```python
from build123d import *

# Parameters (mm, degrees)
SKETCH_1_W          = 28
SKETCH_1_H          = 10
SKETCH_1_R          = 1.65
SKETCH_1_R_2        = 1.6
EXTRUDE_1_DEPTH     = 10
SKETCH_2_R          = 1.65
CUT_EXTRUDE_1_DEPTH = 28
SKETCH_3_W          = 10
SKETCH_3_H          = 10
SKETCH_3_R          = 1.6
CUT_EXTRUDE_2_DEPTH = 7
FILLET_1_R          = 1


with BuildPart() as part:
    # ｽｹｯﾁ1 → ﾎﾞｽ - 押し出し1 (new body)
    with BuildSketch(Plane.XY):
        with Locations((-9, 0)):
            Rectangle(SKETCH_1_W, SKETCH_1_H)
        Circle(SKETCH_1_R, mode=Mode.SUBTRACT)
        with Locations((-18, 0)):
            Circle(SKETCH_1_R_2, mode=Mode.SUBTRACT)
    extrude(amount=EXTRUDE_1_DEPTH)

    # ｽｹｯﾁ2 → ｶｯﾄ - 押し出し1 (cut, through all)
    with BuildSketch(Plane(origin=(0, 5, 0), x_dir=(1, 0, 0), z_dir=(0, 1, 0))):
        with Locations(Location((-7.5, -5, 0), (0, 0, 270))):
            Circle(SKETCH_2_R)
    extrude(amount=-CUT_EXTRUDE_1_DEPTH, mode=Mode.SUBTRACT)

    # ｽｹｯﾁ3 → ｶｯﾄ - 押し出し2 (cut)
    with BuildSketch(Plane(origin=(0, 0, 0), x_dir=(-1, 0, 0), z_dir=(0, 0, -1))):
        with Locations((18, 0)):
            Rectangle(SKETCH_3_W, SKETCH_3_H)
        with Locations((18, 0)):
            Circle(SKETCH_3_R, mode=Mode.SUBTRACT)
    extrude(amount=-CUT_EXTRUDE_2_DEPTH, mode=Mode.SUBTRACT)

    # ﾌｨﾚｯﾄ1
    fillet_1_edges = [part.edges().sort_by_distance(p)[0] for p in [
        (-13, -5, 3.5),
        (-13, 5, 3.5),
        (5, -5, 5),
        (-23, -5, 8.5),
        (-23, 5, 8.5),
        (5, 5, 5),
    ]]
    fillet(fillet_1_edges, radius=FILLET_1_R)


solid = part.part
```
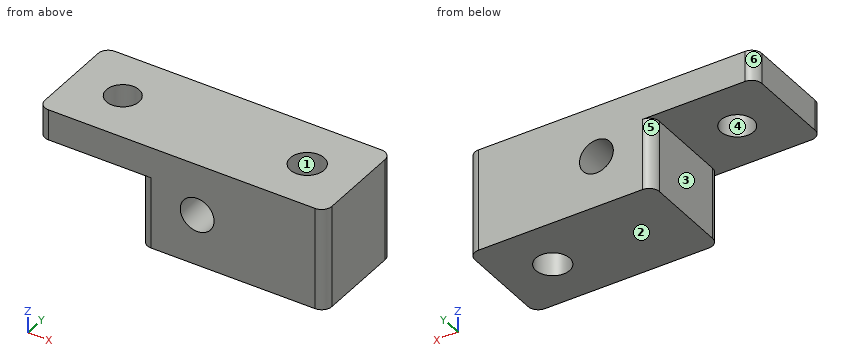
Check sheet for the modelled part. Datum: model origin and axes. Units: mm. Face numbers are marked on the shaded views. A direction names the side the tool comes from. Round coordinates to 2 decimals unless told otherwise and drop trailing zeros. Order: outer loops, then holes, each group sorted by start corner. A loop starts at its lowest first (then second) coordinate and runs counter-clockwise, first axis right, second up. Notation, with made-up numbers: (15, 59) - (51, 59) arc R18 ccw to (51, 90) - close; hole circle Ø6 at (55.25, -32). An arc over 180 degrees is marked (long way). Write item = value, one per line.
Q1. Section check D-D (z = 7.5). Record the boundary of the cut face in (x, y), and give its area (3 significant figures).
Computed:
outline = (-23, -4) arc R1 ccw to (-22, -5) - (4, -5) arc R1 ccw to (5, -4) - (5, 4) arc R1 ccw to (4, 5) - (-22, 5) arc R1 ccw to (-23, 4) - close; hole circle Ø3.2 at (-18, 0); hole circle Ø3.3 at (0, 0)
area = 263 mm^2
Q2. Go/stop test with a flat-tipped pin: pin 1 (3 mm diameter, centred on y = 0, z = 4, fed in from -X). Record where the tip stops, or that it passes through.
Computed:
pin_1 = -13
Q3. Section check A-A (z = 5). Record the boundary of the cut face in (x, y), and give its area (3 significant figures).
Computed:
outline = (-13, -4) arc R1 ccw to (-12, -5) - (-9.15, -5) - (-9.15, 5) - (-12, 5) arc R1 ccw to (-13, 4) - close; (-5.85, -5) - (4, -5) arc R1 ccw to (5, -4) - (5, 4) arc R1 ccw to (4, 5) - (-5.85, 5) - close; hole circle Ø3.3 at (0, 0)
area = 138 mm^2
Q4. Thickness scan on line 1 along X through (y, z) = (-2, 5); line 2 along X through (y, z) = (-1.25, 5); line 3 along Z through (x, y) = (-16.25, -2.5). Record the ranges inside material, lowest first.
Computed:
line_1 = -13 to -9.15, -5.85 to 5
line_2 = -13 to -9.15, -5.85 to -1.08, 1.08 to 5
line_3 = 7 to 10
Q5. Draft check along X on the marked faces 1, 2, 3 and 4. Enter one of: pulls with the +X half, pulls with the -X half, needs draft (parallel to the pull), parting line crosses it, or undercut.
Computed:
face_1 = undercut
face_2 = needs draft
face_3 = pulls with the -X half
face_4 = undercut
Q6. Section check B-B (x = 0). Record the boundary of the cut face in (y, z), and give its area (3 significant figures).
Computed:
outline = (-5, 0) - (-1.65, 0) - (-1.65, 10) - (-5, 10) - close; (1.65, 0) - (5, 0) - (5, 10) - (1.65, 10) - close
area = 67.0 mm^2
Q7. Section check C-C (y = 0). Record the boundary of the cut face in (x, z), and give its area (3 significant figures).
Computed:
outline = (-23, 7) - (-19.6, 7) - (-19.6, 10) - (-23, 10) - close; (-16.4, 7) - (-13, 7) - (-13, 0) - (-1.65, 0) - (-1.65, 10) - (-16.4, 10) - close; (1.65, 0) - (5, 0) - (5, 10) - (1.65, 10) - close; hole circle Ø3.3 at (-7.5, 5)
area = 159 mm^2
Q8. Tool access check on the marked faces 5 and 6. Record the directions out of +Z, -Z, +X, -X, +Y, -Y that give a thin tool (end or side, any length) a straight path to the whole face; none if there is none.
Computed:
face_5 = -Z, -X, +Y
face_6 = +Z, -Z, -X, +Y
